Geometry check sheet. Reference: drawing and pictorial views, mm from the part's lowest x, y, z. A direction names the side the tool comes from. Coordinates: 2 decimals unless noted, no trailing zeros. Write each loop counter-clockwise with the first axis right and the second up, starting at its lowest first coordinate (ties: lowest second). Pieces come first, ordered by that corner, then holes. Notation, with made-up numbers: (72, 17.5) - (103, 17.5) arc R30 cw to (103, 41.5) - close; hole circle Ø10 at (37, -31.75). An arc over 180 degrees is marked (long way). Answer as CSV lines item,"result". Start each with the question number.
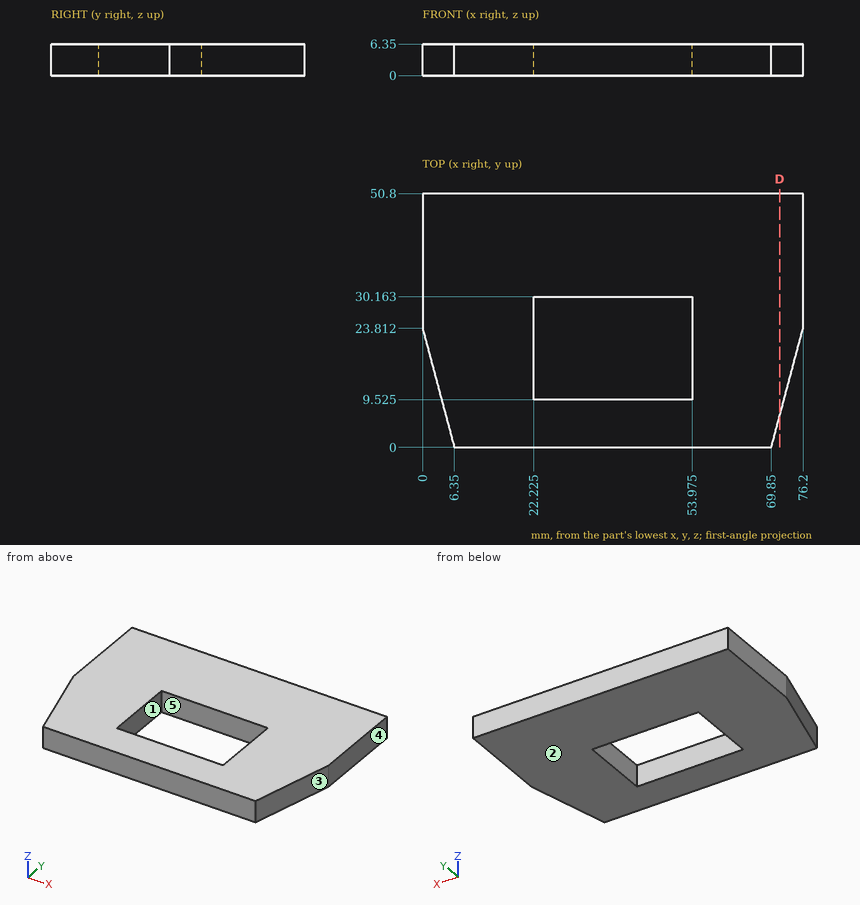
1. Scan lines: line 1 along X through (y, z) = (24, 1.5) (1 decimal); line 2 along Y through (x, z) = (47.5, 1.5) (1 decimal); line 3 along X through (y, z) = (6, 2.5). Record each from-to range of solid material in increasing order. Write a range as from..to.
2. Draft check along Y on the marked faces 3, 4 and 5. Enter one of: pulls with the +Y half, pulls with the -Y half, needs draft (parallel to the pull), parting line crosses it, or undercut.
3. Access from +Z, -Z, +X, -X, +Y, -Y to the whole of each face (thin tool, end or side, straight path). Record for the marked faces 1 and 2.
4. Cross-section at D-D (x = 71.5). Record the cut outline in (y, z), and give its area (3 significant figures).
5. Depth check by flat-ended pin: P1, Ø1.5, axis at x = 68, z = 4, coming from the -Y side; P2, Ø3, axis at y = 18.5, z = 2, coming from the +X side; P3, Ø2, axis at y = 10.5, z = 4.5, coming from the -X side. Enter the tip coordinate at first touch or a pass-through.
Completed:
1,line 1,"x = 0..22.2, 54..76.2"
1,line 2,"y = 0..9.5, 30.2..50.8"
1,line 3,"x = 4.75..71.45"
2,face 3,"pulls with the -Y half"
2,face 4,"needs draft"
2,face 5,"undercut"
3,face 1,"+Z, -Z"
3,face 2,"-Z, +X, -X, +Y, -Y"
4,outline,"(6.19, 0) - (50.8, 0) - (50.8, 6.35) - (6.19, 6.35) - close"
4,area,"283 mm2"
5,P1,"stops at y = 0"
5,P2,"stops at x = 75.18"
5,P3,"stops at x = 3.28"
